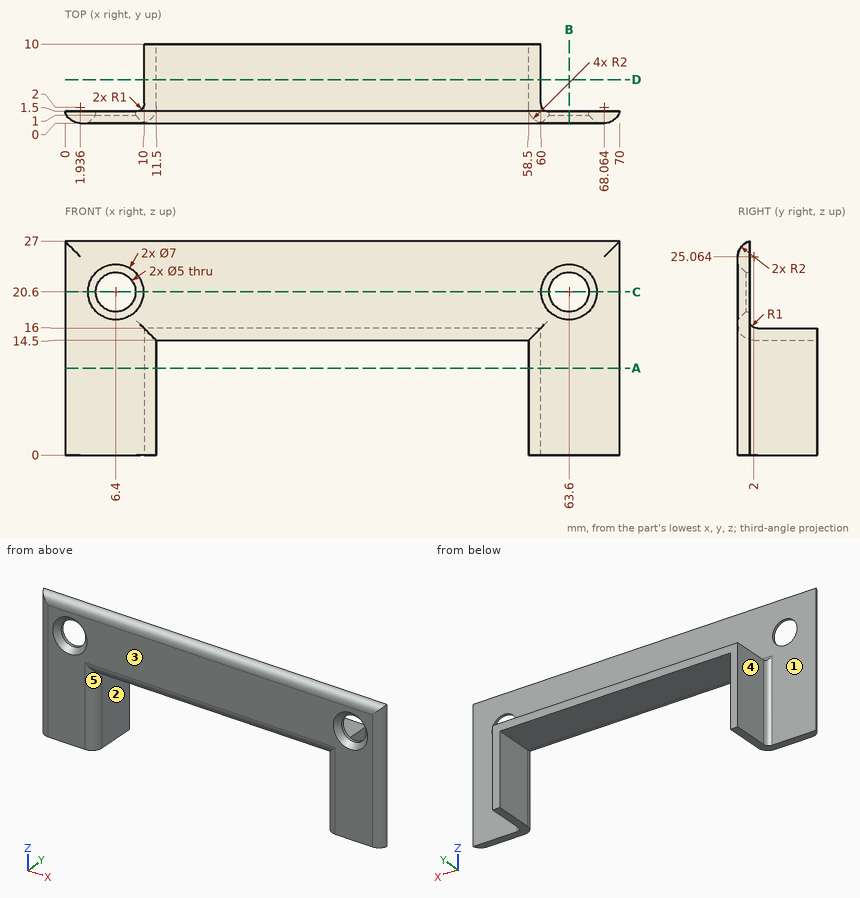
Could you check a few things on this drawing? It's one solid part, dimensions in mm from its lowest x, y, z. A direction names the side the tool comes from. Coordinates: 2 decimals unless noted, no trailing zeros. Order: outer loops, then holes, each group sorted by start corner. A loop starts at its lowest first (then second) coordinate and runs counter-clockwise, first axis right, second up. Notation, with made-up numbers: M -28.5,83 L -2.5,83 A22 cw -2.5,96 Z; hole C 5.25,-19 d5. An arc over 180 degrees is marked long. Use one line per item in the form item = value. Start each with the question number.
1. Suppose I cut it at C-C on z = 20.6. Write out the boundary of the cut face in (x, y).
2. Suppose I cut it at B-B on x = 63.6. Write out the boundary of the cut face in (y, z).
3. Please list where these lines run through material, in increasing order: line 1 (X direction, y = 1.25, z = 20.6); line 2 (X direction, y = 5.5, z = 3.25); line 3 (Z direction, x = 18, y = 7).
4. Suppose I cut it at D-D on y = 5.5. Write out the boundary of the cut face in (x, z).
5. On a 3-axis mill with a long thin cutter (end or side, diameter ignored), from which of +Z, -Z, +X, -X, +Y, -Y can I reach the whole of each face in a straight line? I mean the marked faces 1 and 2. Say none if no direction works.
6. Suppose I cut it at A-A on z = 11. Write out the boundary of the cut face in (x, y).
7. For pin 1 (2.5 mm diameter, centred on y = 7.5, z = 10.5, fed in from -X); pin 2 (4 mm diameter, centred on y = 8, z = 7.5, fed in from +X); pin 3 (4 mm diameter, centred on x = 57.5, y = 6.5, fed in from +Z), each with a flat end and sliding along its axis, tell me the tip position at first contact or that it passes through.
8. We'd pull the mould along X, two halves only. Please class the marked faces 3, 4 and 5: +X half, -X half, draft (parallel to the pull), parting line (faces both ways), or undercut.
Geometry says:
q1.outline = M 0,1.5 A2 ccw 1.94,0 L 2.9,0 L 3.9,1 L 3.9,1.5 Z; M 8.9,1 L 9.9,0 L 60.1,0 L 61.1,1 L 61.1,1.5 L 8.9,1.5 Z; M 66.1,1 L 67.1,0 L 68.06,0 A2 ccw 70,1.5 L 66.1,1.5 Z
q2.outline = M 0,0 L 1.5,0 L 1.5,18.1 L 1,18.1 L 0,17.1 Z; M 0,24.1 L 1,23.1 L 1.5,23.1 L 1.5,27 A2 ccw 0,25.06 Z
q3.line_1 = 0.08 to 3.9, 8.9 to 61.1, 66.1 to 69.92
q3.line_2 = 10 to 11.5, 58.5 to 60
q3.line_3 = 14.5 to 16
q4.outline = M 10,0 L 11.5,0 L 11.5,14.5 L 58.5,14.5 L 58.5,0 L 60,0 L 60,16 L 10,16 Z
q5.face_1 = +Z, +Y
q5.face_2 = -Z, +Y, -Y
q6.outline = M 0,1.5 A2 ccw 1.94,0 L 9.5,0 A2 ccw 11.5,2 L 11.5,10 L 10,10 L 10,2.5 A1 cw 9,1.5 Z; M 58.5,2 A2 ccw 60.5,0 L 68.06,0 A2 ccw 70,1.5 L 61,1.5 A1 cw 60,2.5 L 60,10 L 58.5,10 Z
q7.pin_1 = 10
q7.pin_2 = 60
q7.pin_3 = 16
q8.face_3 = draft
q8.face_4 = -X half
q8.face_5 = undercut
